Geometry: final body of the model. Coordinates: model frame, mm. A direction names the side the tool comes from. Give positions to 0.01 mm unless a question says otherwise; leave off trailing zeros. Write each loop counter-clockwise with the first axis right and the second up, starting at its lowest first coordinate (ties: lowest second). Pieces come first, ordered by that corner, then holes.
Autodesk Inventor part; units mm, degrees
ref_plane "YZ Plane" through (0, 0, 0) normal (1, 0, 0) x (0, 1, 0)
ref_plane "XZ Plane" through (0, 0, 0) normal (0, 1, 0) x (-1, 0, 0)
ref_plane "XY Plane" through (0, 0, 0) normal (0, 0, 1) x (1, 0, 0)
sketch "Sketch1" plane through (0, 0, 0) normal (0, 0, 1) x (1, 0, 0)
  line L0 (0, 0) -> (304.8, 0)
  line L1 (304.8, 0) -> (304.8, 914.4)
  line L2 (304.8, 914.4) -> (0, 914.4)
  line L3 (0, 914.4) -> (0, 0)
  dimension "d0" = 304.8
  dimension "d1" = 914.4
extrude "Extrusion1" add sketch "Sketch1" along normal blind 304.8
sketch "Sketch2" plane through (0, 0, 304.8) normal (0, 0, 1) x (1, 0, 0)
  line L0 (0, 0) -> (304.8, 0)
  line L1 (304.8, 0) -> (304.8, 914.4)
  line L2 (304.8, 914.4) -> (0, 914.4)
  line L3 (0, 914.4) -> (0, 0)
  circle A0 centre (160.2433, 711.2) radius 76.2
  circle A1 centre (160.2433, 457.2) radius 76.2
  circle A2 centre (160.2433, 203.2) radius 76.2
  line L4 (304.8, 914.4) -> (0, 914.4) construction
  line L5 (160.2433, 914.4) -> (160.2433, 895.9675) construction
  dimension "d4" = 152.4
  dimension "d5" = 0
  dimension "d6" = 152.4
  dimension "d7" = 152.4
  dimension "d8" = 254
  dimension "d9" = 254
  dimension "d10" = -203.2
extrude "Extrusion2" cut sketch "Sketch2" against normal blind 152.4 contours A0 | A1 | A2
equation "\"d6\" = d4"
equation "\"d7\" = d4"
equation "\"d9\" = d8"
equation "\"d10\" = -0.5 * d1 + d8"
properties part number "traffic light"
Item 1: Line query: L1, parallel to X at y = 455, z = 232.5; L2, parallel to Y at x = 102, z = 248; L3, parallel to X at y = 182, z = 275.5. Output: solid intervals per line, ascending.
Found:
L1: x = 0 to 84.08, 236.41 to 304.8
L2: y = 0 to 154.07, 252.33 to 408.07, 506.33 to 662.07, 760.33 to 914.4
L3: x = 0 to 87.05, 233.43 to 304.8
Item 2: Section C-C, the plane x = 143. Return the cut outline in (y, z).
Found:
outline: (0, 0) - (914.4, 0) - (914.4, 304.8) - (785.42, 304.8) - (785.42, 152.4) - (636.98, 152.4) - (636.98, 304.8) - (531.42, 304.8) - (531.42, 152.4) - (382.98, 152.4) - (382.98, 304.8) - (277.42, 304.8) - (277.42, 152.4) - (128.98, 152.4) - (128.98, 304.8) - (0, 304.8) - close
Item 3: Reachability of faces 1 (the face through (150, 0, 150)), 2 (the face through (230.63, 174.01, 229.67)) from +Z, -Z, +X, -X, +Y, -Y: full face, straight path, thin tool, end or side. Return the list, or none.
Found:
face 1: +Z, -Z, +X, -X, -Y
face 2: +Z
Item 4: Pull-direction query (Y, two-part tool) for faces 3 (the face through (155, 914.4, 150)), 4 (the face through (159, 204, 152.4)), 5 (the face through (0, 464, 150)); classes: +Y half, -Y half, draft (parallel to the pull), parting line (faces both ways), or undercut.
Found:
face 3: +Y half
face 4: undercut
face 5: draft
Item 5: Pin query (flat end, axial travel): pin 1 Ø4 at (x, y) = (128.5, 438.5) entering from +Z. Return the tip coordinate at first contact, or that it passes through.
Found:
pin 1: stops at z = 152.4
Item 6: Section A-A, the plane z = 273.5. Return the cut outline in (x, y), plus the area to 3 significant figures.
Found:
outline: (0, 0) - (304.8, 0) - (304.8, 914.4) - (0, 914.4) - close; hole circle Ø152.4 at (160.24, 203.2); hole circle Ø152.4 at (160.24, 457.2); hole circle Ø152.4 at (160.24, 711.2)
area: 224,000 mm2
Item 7: Section B-B, the plane y = 457.2. Return the cut outline in (x, z).
Found:
outline: (0, 0) - (304.8, 0) - (304.8, 304.8) - (236.44, 304.8) - (236.44, 152.4) - (84.04, 152.4) - (84.04, 304.8) - (0, 304.8) - close
